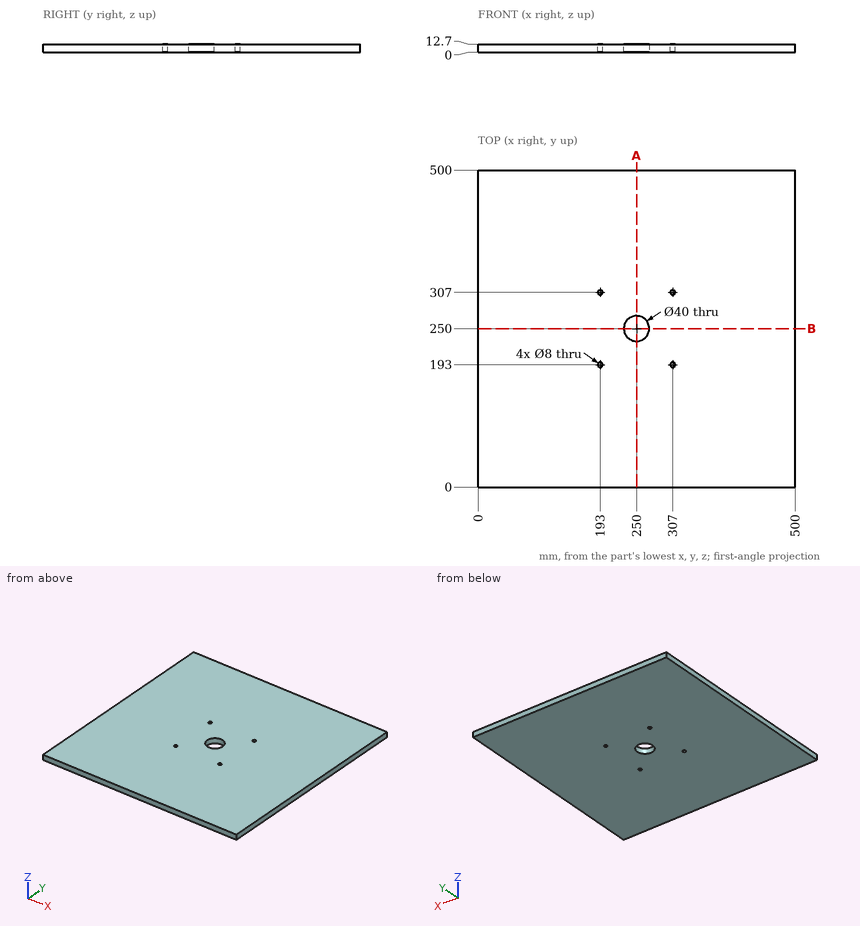
Input: dimensioned drawing with shaded views. Units: mm. Origin: part minimum x, y, z. Round coordinates to 2 decimals unless told otherwise and drop trailing zeros. Loops run counter-clockwise (first coordinate to the right, second up) from the corner with the lowest first, then second, coordinate; pieces in that order, holes last. Notation, with made-up numbers: (12.25, -24.5) -> (63.25, -24.5) arc R18 ccw to (63.25, 3.5) -> close; hole circle Ø9 at (16.5, 32.5). An arc over 180 degrees is marked (long way). One line per item, written item: value.
(1) Material intervals for line 1 (Y direction, x = 193, z = 9); line 2 (Y direction, x = 250, z = 3.75), sorted ascending. Write a range as [from, to].
Geometry check:
line 1: [0, 189], [197, 303], [311, 500]
line 2: [0, 230], [270, 500]
(2) Section A-A (x = 250). Return the cut outline in (y, z).
Geometry check:
outline: (0, 0) -> (230, 0) -> (230, 12.7) -> (0, 12.7) -> close; (270, 0) -> (500, 0) -> (500, 12.7) -> (270, 12.7) -> close
(3) Pin query (flat end, axial travel): pin 1 (5 mm diameter, centred on x = 307, y = 307, fed in from -Z). Return the tip coordinate at first contact, or that it passes through.
Geometry check:
pin 1: through
